Job drawing, mm, ordinate dimensions from the low corner. One solid piece. A direction names the side the tool comes from. Give positions to 0.01 mm unless a question says otherwise; leave off trailing zeros. Loops run counter-clockwise (first coordinate to the right, second up) from the corner with the lowest first, then second, coordinate; pieces in that order, holes last. Notation, with made-up numbers: (32, 40) -> (41, 40) arc R20 ccw to (41, 50) -> close; hole circle Ø9 at (-28.75, 86). An arc over 180 degrees is marked (long way). Answer as a JSON object with one key per item and string values. Group by question number.
Q1. Drop flat-ended pins along their axis: pin 1 (6.5 mm diameter, centred on y = 10, z = 9, fed in from +X); pin 2 (6.5 mm diameter, centred on x = 21, y = 10, fed in from -Z). Give the stop position or say it passes through.
Q2. Two-plate mould, pull along Y, no slides. Class the marked faces 3, 4, 5 and 6: pulls with the +Y half, pulls with the -Y half, needs draft (parallel to the pull), parting line crosses it, or undercut.
Q3. Band-saw the part on D-D, the plane y = 12.5. Write the cut outline in (x, z).
Q4. Band-saw the part on B-B, the plane z = 17. Write the cut outline in (x, y).
Q5. Band-saw the part on C-C, the plane x = 13. Write the cut outline in (y, z).
Q6. Wall check: probe 1 along Y at (x, z) = (21, 28.65); probe 2 along Z at (x, y) = (26.5, 6.5); probe 3 along X at (y, z) = (8.25, 20.25). Give the ranges that are in metal, low to high. Write a range as from..to.
Q7. Band-saw the part on A-A, the plane y = 10. Write the cut outline in (x, z), plus the area to 3 significant figures.
Q8. Tool access for the marked faces 1 and 2: list every direction of +Z, -Z, +X, -X, +Y, -Y with a clear straight run to the whole face (end or side of a thin tool).
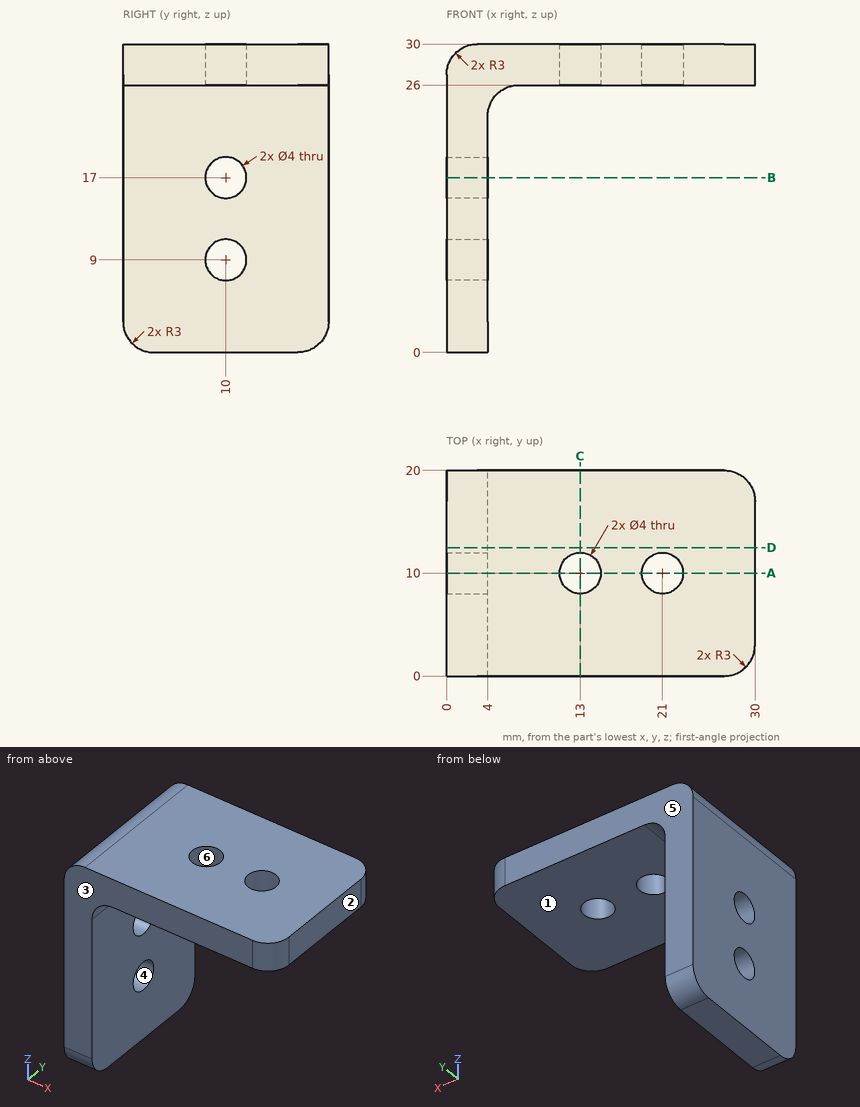
Worked answers:
{
 "1": {"pin 1": "x = 4", "pin 2": "z = 26"},
 "2": {"face 3": "pulls with the -Y half", "face 4": "undercut", "face 5": "pulls with the +Y half", "face 6": "undercut"},
 "3": {"outline": "(0, 0) -> (4, 0) -> (4, 23) arc R3 cw to (7, 26) -> (30, 26) -> (30, 30) -> (3, 30) arc R3 ccw to (0, 27) -> close"},
 "4": {"outline": "(0, 0) -> (4, 0) -> (4, 8) -> (0, 8) -> close; (0, 12) -> (4, 12) -> (4, 20) -> (0, 20) -> close"},
 "5": {"outline": "(0, 26) -> (8, 26) -> (8, 30) -> (0, 30) -> close; (12, 26) -> (20, 26) -> (20, 30) -> (12, 30) -> close"},
 "6": {"probe 1": "0..8, 12..20", "probe 2": "26..30", "probe 3": "0..4"},
 "7": {"outline": "(0, 0) -> (4, 0) -> (4, 7) -> (0, 7) -> close; (0, 11) -> (4, 11) -> (4, 15) -> (0, 15) -> close; (0, 19) -> (4, 19) -> (4, 23) arc R3 cw to (7, 26) -> (11, 26) -> (11, 30) -> (3, 30) arc R3 ccw to (0, 27) -> close; (15, 26) -> (19, 26) -> (19, 30) -> (15, 30) -> close; (23, 26) -> (30, 26) -> (30, 30) -> (23, 30) -> close", "area": "160 mm2"},
 "8": {"face 1": "-Z, +X, +Y, -Y", "face 2": "+Z, -Z, +X, +Y, -Y"}
}
